from build123d import *

# Parameters (mm, degrees)
BOSS_EXTRUDE1_DEPTH = 3.175
FILLET1_R           = 7.62
FILLET2_R           = 2.54
SKETCH4_R           = 1.9685
CUT_EXTRUDE1_DEPTH  = 19.05
FILLET3_R           = 0.508
SKETCH6_R           = 1.778
CUT_EXTRUDE2_DEPTH  = 3.175


with BuildPart() as part:
    # Sketch1 → Boss-Extrude1 (new body)
    with BuildSketch(Plane(origin=(0, 0, 0), x_dir=(1, 0, 0), z_dir=(0, 1, 0))):
        with BuildLine():
            Line((-22.606, 5.715), (22.606, 5.715))
            ThreePointArc((22.606, 5.715), (28.321, 0), (22.606, -5.715))
            Line((22.606, -5.715), (-22.606, -5.715))
            ThreePointArc((-22.606, -5.715), (-28.321, 0), (-22.606, 5.715))
        make_face()
        with BuildLine():
            Line((-5.715, -22.606), (-5.715, 22.606))
            ThreePointArc((-5.715, 22.606), (0, 28.321), (5.715, 22.606))
            Line((5.715, 22.606), (5.715, -22.606))
            ThreePointArc((5.715, -22.606), (0, -28.321), (-5.715, -22.606))
        make_face()
    extrude(amount=BOSS_EXTRUDE1_DEPTH)

    # Fillet1
    fillet1_edges = [part.edges().sort_by_distance(p)[0] for p in [
        (-5.715, 1.5875, -5.715),
        (-5.715, 1.5875, 5.715),
        (5.715, 1.5875, -5.715),
        (5.715, 1.5875, 5.715),
    ]]
    fillet(fillet1_edges, radius=FILLET1_R)

    # Loft1: read off the stored shape, not the designer's step
    # Loft1: loft between two sections, ruled curve by curve
    loft1_from = [
        Edge.make_bspline([(-2.865050686, 3.175, -5.666920201), (-14.198891088, 3.175, 0.063181171), (-8.468789716, 3.175, 11.397021573), (2.865050686, 3.175, 5.666920201), (14.198891088, 3.175, -0.063181171), (8.468789716, 3.175, -11.397021573), (-2.865050686, 3.175, -5.666920201)], [0, 0, 0, 0, 0.5, 0.5, 0.5, 1, 1, 1, 1], 3, [1, 0.333333333, 0.333333333, 1, 0.333333333, 0.333333333, 1]),
    ]
    loft1_to = [
        Edge.make_bspline([(-2.270310983, 22.225, -2.219529914), (-6.709370811, 22.225, 2.321092053), (-2.168748845, 22.225, 6.760151881), (2.270310983, 22.225, 2.219529914), (6.709370811, 22.225, -2.321092053), (2.168748845, 22.225, -6.760151881), (-2.270310983, 22.225, -2.219529914)], [0, 0, 0, 0, 0.5, 0.5, 0.5, 1, 1, 1, 1], 3, [1, 0.333333333, 0.333333333, 1, 0.333333333, 0.333333333, 1]),
    ]
    loft1 = Solid(Shell([*[Face.make_surface_from_curves(loft1_from[k], loft1_to[k]) for k in range(1)], Face(Wire(loft1_from)), Face(Wire(loft1_to))]))
    add(loft1)

    # Fillet2
    fillet2_edges = [part.edges().sort_by_distance(p)[0] for p in [
        (2.865050686, 3.175, 5.666920201),
    ]]
    fillet(fillet2_edges, radius=FILLET2_R)

    # Sketch4 → Cut-Extrude1 (cut)
    with BuildSketch(Plane(origin=(0, 22.225, 0), x_dir=(1, 0, 0), z_dir=(0, 1, 0))):
        with Locations(Location((0, 0, 0), (0, 0, 270))):
            Circle(SKETCH4_R)
    extrude(amount=-CUT_EXTRUDE1_DEPTH, mode=Mode.SUBTRACT)

    # Fillet3
    fillet3_edges = [part.edges().sort_by_distance(p)[0] for p in [
        (2.270310983, 22.225, 2.219529914),
    ]]
    fillet(fillet3_edges, radius=FILLET3_R)

    # Sketch6 → Cut-Extrude2 (cut)
    with BuildSketch(Plane(origin=(0, 3.175, 0), x_dir=(1, 0, 0), z_dir=(0, 1, 0))):
        with Locations(Location((-22.606, 0, 0), (0, 0, 270))):
            Circle(SKETCH6_R)
        with Locations(Location((22.606, 0, 0), (0, 0, 270))):
            Circle(SKETCH6_R)
        with Locations(Location((0, 22.606, 0), (0, 0, 270))):
            Circle(SKETCH6_R)
        with Locations(Location((0, -22.606, 0), (0, 0, 270))):
            Circle(SKETCH6_R)
    extrude(amount=-CUT_EXTRUDE2_DEPTH, mode=Mode.SUBTRACT)


solid = part.part
The model under review builds one solid part; all positions refer to its coordinate system, in mm. A direction names the side the tool comes from. Round coordinates to 2 decimals unless told otherwise and drop trailing zeros. Loops run counter-clockwise (first coordinate to the right, second up) from the corner with the lowest first, then second, coordinate; pieces in that order, holes last. Notation, with made-up numbers: (-15.75, -33.5) -> (27.25, -33.5) arc R21 ccw to (27.25, -25.5) -> close; hole circle Ø7 at (-22.75, 6). An arc over 180 degrees is marked (long way). Return JSON: item names as keys, results as strings.
(1) For line 1 (X direction, y = 2.3, z = 0); line 2 (X direction, y = 1.5, z = -22.5) (3 decimals); line 3 (Y direction, x = -17.5, z = 0) (3 decimals), list the stretches that pass through material, from the lowest coordinate up.
Solved:
{"line 1": "-28.32 to -24.38, -20.83 to 20.83, 24.38 to 28.32", "line 2": "-5.715 to -1.775, 1.775 to 5.715", "line 3": "0 to 3.175"}
(2) For pin 1 (3.5 mm diameter, centred on y = 1.5, z = -18, fed in from -X) (3 decimals); pin 2 (1.6 mm diameter, centred on x = -15.5, y = 1.5, fed in from -Z) (3 decimals); pin 3 (1 mm diameter, centred on y = 4.5, z = 18, fed in from -X); pin 4 (1 mm diameter, centred on y = 2, z = -20, fed in from +X) (3 decimals), all flat-tipped, find the tip position at first contact; note any pin that passes through.
Solved:
{"pin 1": "x = -5.715", "pin 2": "z = -5.715", "pin 3": "through", "pin 4": "x = 5.715"}
(3) For faces 1 (the flat face through (0, 3.175, 0)), 2 (the flat face through (18, 2, -5.715)), 3 (the flat face through (-18, 2, 5.715)), 4 (the flat face through (18, 2, 5.715)), list the 3-axis set-ups (+Z, -Z, +X, -X, +Y, -Y) from which the entire face can be reached by the end or side of a thin tool; tool diameter is ignored.
Solved:
{"face 1": "+Y", "face 2": "-Z, +X, +Y, -Y", "face 3": "+Z, -X, +Y, -Y", "face 4": "+Z, +X, +Y, -Y"}
(4) Add section A-A on z = 19. Write out the cut boundary in (x, y) (3 decimals).
Solved:
{"outline": "(-5.715, 0) -> (5.715, 0) -> (5.715, 3.175) -> (-5.715, 3.175) -> close"}
(5) Add section B-B on x = 20. Write out the cut boundary in (y, z) (3 decimals).
Solved:
{"outline": "(0, -5.715) -> (3.175, -5.715) -> (3.175, 5.715) -> (0, 5.715) -> close"}
(6) Add section C-C on x = 0. State how many separate pieces and enclosed holes the cut face has, plus the area to 3 significant figures.
Solved:
{"separate pieces": "3", "enclosed holes": "0", "area": "264 mm2"}
